Build history of the part. All positions in model axes, mm. Face numbers are marked on the shaded views. Round coordinates to 2 decimals unless told otherwise and drop trailing zeros. Loops run counter-clockwise (first coordinate to the right, second up) from the corner with the lowest first, then second, coordinate; pieces in that order, holes last. Notation, with made-up numbers: (81.25, 76) - (117.25, 76) arc R23 cw to (117.25, 101) - close; hole circle Ø1 at (66.5, -4). An arc over 180 degrees is marked (long way). Use a Markdown table: item, result.
from build123d import *

# Parameters (mm, degrees)
BOSS_EXTRUDE1_DEPTH                               = 25.4
CHAMFER1_SIZE                                     = 1.27
CSK_FOR_8_FLAT_HEAD_MACHINE_SCREW_100_D           = 4.9149
CSK_FOR_8_FLAT_HEAD_MACHINE_SCREW_100_CSINK_D     = 8.4328
CSK_FOR_8_FLAT_HEAD_MACHINE_SCREW_100_CSINK_ANGLE = 100


with BuildPart() as part:
    # Sketch1 → Boss-Extrude1 (new body)
    with BuildSketch(Plane.XY):
        with BuildLine():
            Line((-6.35, -3.175), (-6.35, 3.175))
            ThreePointArc((-6.35, 3.175), (0, 9.525), (6.35, 3.175))
            Line((6.35, 3.175), (6.35, -3.175))
            ThreePointArc((6.35, -3.175), (0, -9.525), (-6.35, -3.175))
        make_face()
    extrude(amount=BOSS_EXTRUDE1_DEPTH)

    # Chamfer1
    chamfer1_edges = [part.edges().sort_by_distance(p)[0] for p in [
        (0, 9.525, 25.4),
        (-6.35, 0, 25.4),
        (0, -9.525, 25.4),
        (-6.35, 0, 0),
        (0, 9.525, 0),
        (6.35, 0, 0),
        (0, -9.525, 0),
        (6.35, 0, 25.4),
    ]]
    chamfer(chamfer1_edges, length=CHAMFER1_SIZE)

    # CSK for #8 Flat Head Machine Screw (100)1 (through all)
    with Locations(Plane.XY.offset(25.4)):
        with Locations((0, 0)):
            CounterSinkHole(CSK_FOR_8_FLAT_HEAD_MACHINE_SCREW_100_D / 2, CSK_FOR_8_FLAT_HEAD_MACHINE_SCREW_100_CSINK_D / 2, counter_sink_angle=CSK_FOR_8_FLAT_HEAD_MACHINE_SCREW_100_CSINK_ANGLE)


solid = part.part
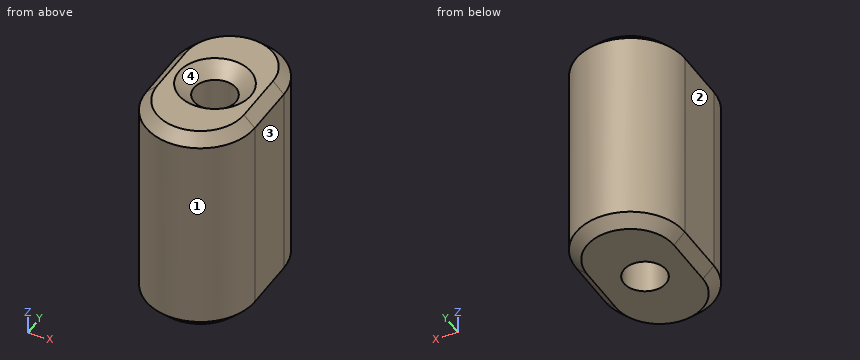
Q1. Cut at C-C, the plane z = 13.5. List the corners of the cut face in (x, y) (3 decimals), plus the area to 3 significant figures.
Results found:
| item | result |
|---|---|
| outline | (-6.35, -3.175) arc R6.35 ccw to (6.35, -3.175) - (6.35, 3.175) arc R6.35 ccw to (-6.35, 3.175) - close; hole circle Ø4.915 at (0, 0) |
| area | 188 mm2 |
Q2. Drop a flat-ended pin along its axis: pin 1 (1.5 mm diameter, centred on y = 5, z = 15, fed in from -X). Give the stop position or say it passes through.
Results found:
| item | result |
|---|---|
| pin 1 | stops at x = -6.26 |
Q3. Pull direction X, two halves, no side cores. Call the marked faces 1, 2, 3 and 4: pulls with the +X half, pulls with the -X half, needs draft (parallel to the pull), parting line crosses it, or undercut.
Results found:
| item | result |
|---|---|
| face 1 | parting line crosses it |
| face 2 | pulls with the -X half |
| face 3 | pulls with the +X half |
| face 4 | undercut |
Q4. Cut at B-B, the plane y = 0. List the corners of the cut face in (x, z), plus the area to 3 significant figures.
Results found:
| item | result |
|---|---|
| outline | (-6.35, 1.27) - (-5.08, 0) - (-2.46, 0) - (-2.46, 23.92) - (-4.22, 25.4) - (-5.08, 25.4) - (-6.35, 24.13) - close; (2.46, 0) - (5.08, 0) - (6.35, 1.27) - (6.35, 24.13) - (5.08, 25.4) - (4.22, 25.4) - (2.46, 23.92) - close |
| area | 192 mm2 |
Q5. Cut at A-A, the plane x = 0. List the corners of the cut face in (y, z) (3 decimals), plus the area to 3 significant figures.
Results found:
| item | result |
|---|---|
| outline | (-9.525, 1.27) - (-8.255, 0) - (-2.457, 0) - (-2.457, 23.924) - (-4.216, 25.4) - (-8.255, 25.4) - (-9.525, 24.13) - close; (2.457, 0) - (8.255, 0) - (9.525, 1.27) - (9.525, 24.13) - (8.255, 25.4) - (4.216, 25.4) - (2.457, 23.924) - close |
| area | 353 mm2 |
Q6. Probe line 1 (Y direction, x = 0, z = 10.75) (3 decimals); line 2 (X direction, y = 0, z = 14.5); line 3 (Y direction, x = -1, z = 11.5). List the from-to ranges inside material, lowest first.
Results found:
| item | result |
|---|---|
| line 1 | y = -9.525 to -2.457, 2.457 to 9.525 |
| line 2 | x = -6.35 to -2.46, 2.46 to 6.35 |
| line 3 | y = -9.45 to -2.24, 2.24 to 9.45 |
